from build123d import *

# Parameters (mm, degrees)
F0_R      = 3.5
F1_DEPTH  = 2
F3_DEPTH  = 5.1
F4_R      = 2.6
F5_R      = 5
F6_T      = -1.6
F8_DEPTH  = 2
F9_R      = 3.5
F10_DEPTH = 29.2431356237


with BuildPart() as f1:
    # F0 (on Top) → F1 (new body)
    with BuildSketch(Plane.XY):
        with BuildLine():
            Line((-7.0710678119, 21.2132034356), (-21.2132034356, 7.0710678119))
            ThreePointArc((-21.2132034356, 7.0710678119), (-24.1421356237, 0), (-21.2132034356, -7.0710678119))
            Line((-21.2132034356, -7.0710678119), (-7.0710678119, -21.2132034356))
            ThreePointArc((-7.0710678119, -21.2132034356), (0, -24.1421356237), (7.0710678119, -21.2132034356))
            Line((7.0710678119, -21.2132034356), (21.2132034356, -7.0710678119))
            ThreePointArc((21.2132034356, -7.0710678119), (24.1421356237, 0), (21.2132034356, 7.0710678119))
            Line((21.2132034356, 7.0710678119), (7.0710678119, 21.2132034356))
            ThreePointArc((7.0710678119, 21.2132034356), (0, 24.1421356237), (-7.0710678119, 21.2132034356))
        make_face()
        with Locations((0, -16.9705627485)):
            Circle(F0_R, mode=Mode.SUBTRACT)
        with Locations((-16.9705627485, 0)):
            Circle(F0_R, mode=Mode.SUBTRACT)
        with Locations((16.9705627485, 0)):
            Circle(F0_R, mode=Mode.SUBTRACT)
        with Locations((0, 16.9705627485)):
            Circle(F0_R, mode=Mode.SUBTRACT)
    extrude(amount=F1_DEPTH)



with BuildPart() as f3:
    # F2 (on Front) → F3 (new body, symmetric)
    with BuildSketch(Plane.XZ):
        Polygon((-300, 2), (300, 2), (272.3112537903, 49.9583152331), (122.3112537903, 49.9583152331), (108.4668806854, 25.9791576166), (0, 25.9791576166), (-108.4668806854, 25.9791576166), (-122.3112537903, 49.9583152331), (-272.3112537903, 49.9583152331), align=None)
    extrude(amount=F3_DEPTH, both=True)

    # F4
    f4_edges = [f3.edges().sort_by_distance(p)[0] for p in [
        (0, -5.1, 2),
        (0, 5.1, 2),
    ]]
    fillet(f4_edges, radius=F4_R)

    # F5
    f5_edges = [f3.edges().sort_by_distance(p)[0] for p in [
        (-272.311254, 0, 49.958315),
        (-122.311254, 0, 49.958315),
        (-108.466881, 0, 25.979158),
        (122.311254, 0, 49.958315),
        (108.466881, 0, 25.979158),
        (272.311254, 0, 49.958315),
    ]]
    fillet(f5_edges, radius=F5_R)

    # F6
    f6_openings = [f3.faces().sort_by_distance(p)[0] for p in [
        (-286.796795, 0, 24.868623),
        (-271.924502, 0, 49.288442),
        (-197.311254, 0, 49.958315),
        (0, 0, 25.979158),
        (-108.080129, 0, 26.649031),
        (-115.389067, 0, 37.968736),
        (-122.698005, 0, 49.288442),
        (108.080129, 0, 26.649031),
        (115.389067, 0, 37.968736),
        (122.698005, 0, 49.288442),
        (197.311254, 0, 49.958315),
        (271.924502, 0, 49.288442),
        (286.796795, 0, 24.868623),
    ]]
    offset(amount=F6_T, openings=f6_openings)


with BuildPart() as f1_1:
    add(f1.part)

    add(f3.part)  # F8 merges F3
    # F7 (on face) → F8 (join, through all)
    with BuildSketch(Plane(origin=(0, 0, 0), x_dir=(1, 0, 0), z_dir=(0, 0, -1))):
        with BuildLine():
            Line((-298, -5.1), (298, -5.1))
            ThreePointArc((298, -5.1), (299.4142135624, -4.5142135624), (300, -3.1))
            Line((300, -3.1), (300, 3.1))
            ThreePointArc((300, 3.1), (299.4142135624, 4.5142135624), (298, 5.1))
            Line((298, 5.1), (-298, 5.1))
            ThreePointArc((-298, 5.1), (-299.4142135624, 4.5142135624), (-300, 3.1))
            Line((-300, 3.1), (-300, -3.1))
            ThreePointArc((-300, -3.1), (-299.4142135624, -4.5142135624), (-298, -5.1))
        make_face()
    extrude(amount=-F8_DEPTH)

    # F9 (on face) → F10 (cut, through all)
    with BuildSketch(Plane.XZ.offset(5.1)):
        with Locations((-197.5, 24.9583152331)):
            Circle(F9_R)
        with Locations((197.5, 24.9583152331)):
            Circle(F9_R)
    extrude(amount=-F10_DEPTH, mode=Mode.SUBTRACT)


solid = f1_1.part
Here's how the part is built. I have some questions about the finished solid (model axes, mm). A direction names the side the tool comes from. Coordinates: 2 decimals unless noted, no trailing zeros. Write each loop counter-clockwise with the first axis right and the second up, starting at its lowest first coordinate (ties: lowest second). Pieces come first, ordered by that corner, then holes.
Item 1: If I drill on line 1 (Y direction, x = 0, z = 0.6); line 2 (Z direction, x = 197.5, y = 4.6); line 3 (Z direction, x = -197.5, y = -4), over which ranges is the centre line in solid material (lowest first)?
Item 2: If we mould it in two halves opening along Y, with no side actions, what happens to faces 5 (the flat face through (-4, 3.5, 23)), 6 (the flat face through (-14.043, 14.241, 0.986)), 7 (the flat face through (-287.79, -3.8, 23.15))? For each: +Y half, -Y half, draft (parallel to the pull), parting line (faces both ways), or undercut.
Item 3: I want a section at A-A on x = 258.5. Write out the boundary of the cut face in (y, z).
Item 4: Will these pins go through, and if not, where does the flat tip stop? pin 1 (3 mm diameter, centred on x = 185, z = 32, fed in from -Y); pin 2 (4 mm diameter, centred on y = -5, z = 14.5, fed in from -X); pin 3 (8 mm diameter, centred on x = 197.5, z = 24.96, fed in from +Y); pin 4 (12 mm diameter, centred on x = -191, y = 2, fed in from -Z).
Item 5: On a 3-axis mill with a long thin cutter (end or side, diameter ignored), from which of +Z, -Z, +X, -X, +Y, -Y can I reach the whole of each face in a straight line? I mean faces 1 (the flat face through (-1, 5, 2)), 2 (the flat face through (-115.312, 4.289, 37.836)), 3 (the flat face through (-14.241, -14.043, 0.986)), 4 (the flat face through (-4, -3.5, 23)). Say none if no direction works.
Item 6: I want a section at B-B on z = 33.5. Write out the boundary of the cut face in (x, y), and give its area (3 significant figures).
Item 7: I want a section at C-C on x = -115. Write out the boundary of the cut face in (y, z).
Findings below:
1. line 1: y = -24.14 to -20.47, -13.47 to 13.47, 20.47 to 24.14
1. line 2: z = 0 to 2, 3.07 to 21.46, 28.46 to 49.96
1. line 3: z = 0 to 2, 2.48 to 21.46, 28.46 to 49.96
2. face 5: undercut
2. face 6: +Y half
2. face 7: draft
3. outline: (-5.1, 0) - (5.1, 0) - (5.1, 2) - (2.5, 2) arc R2.6 ccw to (5.1, 4.6) - (5.1, 49.96) - (3.5, 49.96) - (3.5, 4.6) arc R1 cw to (2.5, 3.6) - (-2.5, 3.6) arc R1 cw to (-3.5, 4.6) - (-3.5, 49.96) - (-5.1, 49.96) - (-5.1, 4.6) arc R2.6 ccw to (-2.5, 2) - (-5.1, 2) - close
4. pin 1: stops at y = -5.1
4. pin 2: stops at x = -293.94
4. pin 3: stops at y = 5.1
4. pin 4: stops at z = 0
5. face 1: none
5. face 2: +Z, +Y, -Y
5. face 3: +Z, -Z, -X, -Y
5. face 4: +Z, +X, -X
6. outline: (-281.81, -5.1) - (-112.81, -5.1) - (-112.81, -3.5) - (-281.81, -3.5) - close; (-281.81, 3.5) - (-112.81, 3.5) - (-112.81, 5.1) - (-281.81, 5.1) - close; (112.81, -5.1) - (281.81, -5.1) - (281.81, -3.5) - (112.81, -3.5) - close; (112.81, 3.5) - (281.81, 3.5) - (281.81, 5.1) - (112.81, 5.1) - close
6. area: 1,080 mm2
7. outline: (-5.1, 0) - (5.1, 0) - (5.1, 2) - (2.5, 2) arc R2.6 ccw to (5.1, 4.6) - (5.1, 37.29) - (3.5, 37.29) - (3.5, 4.6) arc R1 cw to (2.5, 3.6) - (-2.5, 3.6) arc R1 cw to (-3.5, 4.6) - (-3.5, 37.29) - (-5.1, 37.29) - (-5.1, 4.6) arc R2.6 ccw to (-2.5, 2) - (-5.1, 2) - close
